from build123d import *

# Parameters (mm, degrees)
ESQUISSE1_W             = 43
ESQUISSE1_H             = 80
BOSS_EXTRU_1_DEPTH      = 5
ESQUISSE2_W             = 5
ESQUISSE2_H             = 80
BOSS_EXTRU_2_DEPTH      = 38.5
ENL_V_MAT_EXTRU_1_REACH = 84.692
ESQUISSE3_R             = 1.75
ESQUISSE4_W             = 5
ESQUISSE4_H             = 80
BOSS_EXTRU_3_DEPTH      = 20
ENL_V_MAT_EXTRU_2_REACH = 82.206
ESQUISSE5_R             = 2.75
ENL_V_MAT_EXTRU_3_REACH = 80.13
ESQUISSE6_R             = 1.5
BOSS_EXTRU_4_DEPTH      = 80
ENL_V_MAT_EXTRU_4_REACH = 82.206
ESQUISSE8_R             = 6
CHANFREIN2_SIZE         = 8.5
CHANFREIN2_SIZE2        = 10


with BuildPart() as part:
    # Esquisse1 → Boss.-Extru.1 (new body)
    with BuildSketch(Plane.XY):
        with Locations((-11.896872358, -15.648351648)):
            Rectangle(ESQUISSE1_W, ESQUISSE1_H)
    extrude(amount=BOSS_EXTRU_1_DEPTH)

    # Esquisse2 → Boss.-Extru.2 (add)
    with BuildSketch(Plane(origin=(0, 0, 5), x_dir=(-1, 0, 0), z_dir=(0, 0, -1))):
        with Locations((-7.103127642, -15.648351648)):
            Rectangle(ESQUISSE2_W, ESQUISSE2_H)
    extrude(amount=-BOSS_EXTRU_2_DEPTH)

    # Esquisse3 → Enlèv. mat.-Extru.1 (cut, up to next)
    with BuildSketch(Plane(origin=(9.603127642, 0, 0), x_dir=(0, 0, -1), z_dir=(1, 0, 0)), mode=Mode.PRIVATE) as enl_v_mat_extru_1_sk1:
        with Locations(Location((-40, -52.148351648, 0), (0, 0, 90))):
            Circle(ESQUISSE3_R)
    enl_v_mat_extru_1_tool1 = extrude(enl_v_mat_extru_1_sk1.sketch, amount=-ENL_V_MAT_EXTRU_1_REACH, mode=Mode.PRIVATE) & part.part
    # Esquisse3 → Enlèv. mat.-Extru.1 (cut, up to next)
    with BuildSketch(Plane(origin=(9.603127642, 0, 0), x_dir=(0, 0, -1), z_dir=(1, 0, 0)), mode=Mode.PRIVATE) as enl_v_mat_extru_1_sk2:
        with Locations(Location((-40, -32.148351648, 0), (0, 0, 90))):
            Circle(ESQUISSE3_R)
    enl_v_mat_extru_1_tool2 = extrude(enl_v_mat_extru_1_sk2.sketch, amount=-ENL_V_MAT_EXTRU_1_REACH, mode=Mode.PRIVATE) & part.part
    # Esquisse3 → Enlèv. mat.-Extru.1 (cut, up to next)
    with BuildSketch(Plane(origin=(9.603127642, 0, 0), x_dir=(0, 0, -1), z_dir=(1, 0, 0)), mode=Mode.PRIVATE) as enl_v_mat_extru_1_sk3:
        with Locations(Location((-20, -32.148351648, 0), (0, 0, 90))):
            Circle(ESQUISSE3_R)
    enl_v_mat_extru_1_tool3 = extrude(enl_v_mat_extru_1_sk3.sketch, amount=-ENL_V_MAT_EXTRU_1_REACH, mode=Mode.PRIVATE) & part.part
    # Esquisse3 → Enlèv. mat.-Extru.1 (cut, up to next)
    with BuildSketch(Plane(origin=(9.603127642, 0, 0), x_dir=(0, 0, -1), z_dir=(1, 0, 0)), mode=Mode.PRIVATE) as enl_v_mat_extru_1_sk4:
        with Locations(Location((-20, -52.148351648, 0), (0, 0, 90))):
            Circle(ESQUISSE3_R)
    enl_v_mat_extru_1_tool4 = extrude(enl_v_mat_extru_1_sk4.sketch, amount=-ENL_V_MAT_EXTRU_1_REACH, mode=Mode.PRIVATE) & part.part
    # Esquisse3 → Enlèv. mat.-Extru.1 (cut, up to next)
    with BuildSketch(Plane(origin=(9.603127642, 0, 0), x_dir=(0, 0, -1), z_dir=(1, 0, 0)), mode=Mode.PRIVATE) as enl_v_mat_extru_1_sk5:
        with Locations(Location((-40, 0.851648352, 0), (0, 0, 90))):
            Circle(ESQUISSE3_R)
    enl_v_mat_extru_1_tool5 = extrude(enl_v_mat_extru_1_sk5.sketch, amount=-ENL_V_MAT_EXTRU_1_REACH, mode=Mode.PRIVATE) & part.part
    # Esquisse3 → Enlèv. mat.-Extru.1 (cut, up to next)
    with BuildSketch(Plane(origin=(9.603127642, 0, 0), x_dir=(0, 0, -1), z_dir=(1, 0, 0)), mode=Mode.PRIVATE) as enl_v_mat_extru_1_sk6:
        with Locations(Location((-40, 20.851648352, 0), (0, 0, 90))):
            Circle(ESQUISSE3_R)
    enl_v_mat_extru_1_tool6 = extrude(enl_v_mat_extru_1_sk6.sketch, amount=-ENL_V_MAT_EXTRU_1_REACH, mode=Mode.PRIVATE) & part.part
    # Esquisse3 → Enlèv. mat.-Extru.1 (cut, up to next)
    with BuildSketch(Plane(origin=(9.603127642, 0, 0), x_dir=(0, 0, -1), z_dir=(1, 0, 0)), mode=Mode.PRIVATE) as enl_v_mat_extru_1_sk7:
        with Locations(Location((-20, 20.851648352, 0), (0, 0, 90))):
            Circle(ESQUISSE3_R)
    enl_v_mat_extru_1_tool7 = extrude(enl_v_mat_extru_1_sk7.sketch, amount=-ENL_V_MAT_EXTRU_1_REACH, mode=Mode.PRIVATE) & part.part
    # Esquisse3 → Enlèv. mat.-Extru.1 (cut, up to next)
    with BuildSketch(Plane(origin=(9.603127642, 0, 0), x_dir=(0, 0, -1), z_dir=(1, 0, 0)), mode=Mode.PRIVATE) as enl_v_mat_extru_1_sk8:
        with Locations(Location((-20, 0.851648352, 0), (0, 0, 90))):
            Circle(ESQUISSE3_R)
    enl_v_mat_extru_1_tool8 = extrude(enl_v_mat_extru_1_sk8.sketch, amount=-ENL_V_MAT_EXTRU_1_REACH, mode=Mode.PRIVATE) & part.part
    add(enl_v_mat_extru_1_tool1.solids().sort_by_distance((9.603128, -52.148352, 40))[0], mode=Mode.SUBTRACT)
    add(enl_v_mat_extru_1_tool2.solids().sort_by_distance((9.603128, -32.148352, 40))[0], mode=Mode.SUBTRACT)
    add(enl_v_mat_extru_1_tool3.solids().sort_by_distance((9.603128, -32.148352, 20))[0], mode=Mode.SUBTRACT)
    add(enl_v_mat_extru_1_tool4.solids().sort_by_distance((9.603128, -52.148352, 20))[0], mode=Mode.SUBTRACT)
    add(enl_v_mat_extru_1_tool5.solids().sort_by_distance((9.603128, 0.851648, 40))[0], mode=Mode.SUBTRACT)
    add(enl_v_mat_extru_1_tool6.solids().sort_by_distance((9.603128, 20.851648, 40))[0], mode=Mode.SUBTRACT)
    add(enl_v_mat_extru_1_tool7.solids().sort_by_distance((9.603128, 20.851648, 20))[0], mode=Mode.SUBTRACT)
    add(enl_v_mat_extru_1_tool8.solids().sort_by_distance((9.603128, 0.851648, 20))[0], mode=Mode.SUBTRACT)

    # Esquisse4 → Boss.-Extru.3 (add)
    with BuildSketch(Plane(origin=(0, 0, 0), x_dir=(-1, 0, 0), z_dir=(0, 0, -1))):
        with Locations((30.896872358, -15.648351648)):
            Rectangle(ESQUISSE4_W, ESQUISSE4_H)
    extrude(amount=BOSS_EXTRU_3_DEPTH)

    # Esquisse5 → Enlèv. mat.-Extru.2 (cut, up to next)
    with BuildSketch(Plane(origin=(-28.396872358, 0, 0), x_dir=(0, 0, -1), z_dir=(1, 0, 0)), mode=Mode.PRIVATE) as enl_v_mat_extru_2_sk1:
        with Locations(Location((10, 14.351648352, 0), (0, 0, 90))):
            Circle(ESQUISSE5_R)
    enl_v_mat_extru_2_tool1 = extrude(enl_v_mat_extru_2_sk1.sketch, amount=-ENL_V_MAT_EXTRU_2_REACH, mode=Mode.PRIVATE) & part.part
    # Esquisse5 → Enlèv. mat.-Extru.2 (cut, up to next)
    with BuildSketch(Plane(origin=(-28.396872358, 0, 0), x_dir=(0, 0, -1), z_dir=(1, 0, 0)), mode=Mode.PRIVATE) as enl_v_mat_extru_2_sk2:
        with Locations(Location((10, -5.648351648, 0), (0, 0, 90))):
            Circle(ESQUISSE5_R)
    enl_v_mat_extru_2_tool2 = extrude(enl_v_mat_extru_2_sk2.sketch, amount=-ENL_V_MAT_EXTRU_2_REACH, mode=Mode.PRIVATE) & part.part
    # Esquisse5 → Enlèv. mat.-Extru.2 (cut, up to next)
    with BuildSketch(Plane(origin=(-28.396872358, 0, 0), x_dir=(0, 0, -1), z_dir=(1, 0, 0)), mode=Mode.PRIVATE) as enl_v_mat_extru_2_sk3:
        with Locations(Location((10, -25.648351648, 0), (0, 0, 90))):
            Circle(ESQUISSE5_R)
    enl_v_mat_extru_2_tool3 = extrude(enl_v_mat_extru_2_sk3.sketch, amount=-ENL_V_MAT_EXTRU_2_REACH, mode=Mode.PRIVATE) & part.part
    # Esquisse5 → Enlèv. mat.-Extru.2 (cut, up to next)
    with BuildSketch(Plane(origin=(-28.396872358, 0, 0), x_dir=(0, 0, -1), z_dir=(1, 0, 0)), mode=Mode.PRIVATE) as enl_v_mat_extru_2_sk4:
        with Locations(Location((10, -45.648351648, 0), (0, 0, 90))):
            Circle(ESQUISSE5_R)
    enl_v_mat_extru_2_tool4 = extrude(enl_v_mat_extru_2_sk4.sketch, amount=-ENL_V_MAT_EXTRU_2_REACH, mode=Mode.PRIVATE) & part.part
    add(enl_v_mat_extru_2_tool1.solids().sort_by_distance((-28.396872, 14.351648, -10))[0], mode=Mode.SUBTRACT)
    add(enl_v_mat_extru_2_tool2.solids().sort_by_distance((-28.396872, -5.648352, -10))[0], mode=Mode.SUBTRACT)
    add(enl_v_mat_extru_2_tool3.solids().sort_by_distance((-28.396872, -25.648352, -10))[0], mode=Mode.SUBTRACT)
    add(enl_v_mat_extru_2_tool4.solids().sort_by_distance((-28.396872, -45.648352, -10))[0], mode=Mode.SUBTRACT)

    # Esquisse6 → Enlèv. mat.-Extru.3 (cut, up to next)
    with BuildSketch(Plane(origin=(0, 0, 0), x_dir=(-1, 0, 0), z_dir=(0, 0, -1)), mode=Mode.PRIVATE) as enl_v_mat_extru_3_sk1:
        with Locations((18.396872358, -45.648351648)):
            Circle(ESQUISSE6_R)
    enl_v_mat_extru_3_tool1 = extrude(enl_v_mat_extru_3_sk1.sketch, amount=-ENL_V_MAT_EXTRU_3_REACH, mode=Mode.PRIVATE) & part.part
    add(enl_v_mat_extru_3_tool1.solids().sort_by_distance((-18.396872, -45.648352, 0))[0], mode=Mode.SUBTRACT)

    # Esquisse7 → Boss.-Extru.4 (add)
    with BuildSketch(Plane(origin=(0, 24.351648352, 0), x_dir=(1, 0, 0), z_dir=(0, 1, 0))):
        Polygon((9.603127642, 0), (-28.396872358, 20), (-28.396872358, 14.349760381), (-1.132327635, 0), align=None)
    extrude(amount=-BOSS_EXTRU_4_DEPTH)

    # Enlèv. mat.-Extru.4: up to this plane
    enl_v_mat_extru_4_end = Plane(origin=(9.603127642, -98.590172756, 0), z_dir=(0.46574643283262246, 0, -0.8849182223819824))
    # Esquisse8 → Enlèv. mat.-Extru.4 (cut, up to the surface)
    with BuildSketch(Plane(origin=(-28.396872358, 0, 0), x_dir=(0, 0, -1), z_dir=(1, 0, 0)), mode=Mode.PRIVATE) as enl_v_mat_extru_4_sk1:
        with Locations(Location((10, -45.648351648, 0), (0, 0, 316.465525683))):
            Circle(ESQUISSE8_R)
    enl_v_mat_extru_4_tool1 = split(extrude(enl_v_mat_extru_4_sk1.sketch, amount=ENL_V_MAT_EXTRU_4_REACH, mode=Mode.PRIVATE), bisect_by=enl_v_mat_extru_4_end, keep=Keep.BOTH, mode=Mode.PRIVATE)
    add(enl_v_mat_extru_4_tool1.solids().sort_by_distance((-28.396872, -45.648352, -10))[0], mode=Mode.SUBTRACT)
    # Esquisse8 → Enlèv. mat.-Extru.4 (cut, up to the surface)
    with BuildSketch(Plane(origin=(-28.396872358, 0, 0), x_dir=(0, 0, -1), z_dir=(1, 0, 0)), mode=Mode.PRIVATE) as enl_v_mat_extru_4_sk2:
        with Locations(Location((10, -25.648351648, 0), (0, 0, 316.465525683))):
            Circle(ESQUISSE8_R)
    enl_v_mat_extru_4_tool2 = split(extrude(enl_v_mat_extru_4_sk2.sketch, amount=ENL_V_MAT_EXTRU_4_REACH, mode=Mode.PRIVATE), bisect_by=enl_v_mat_extru_4_end, keep=Keep.BOTH, mode=Mode.PRIVATE)
    add(enl_v_mat_extru_4_tool2.solids().sort_by_distance((-28.396872, -25.648352, -10))[0], mode=Mode.SUBTRACT)
    # Esquisse8 → Enlèv. mat.-Extru.4 (cut, up to the surface)
    with BuildSketch(Plane(origin=(-28.396872358, 0, 0), x_dir=(0, 0, -1), z_dir=(1, 0, 0)), mode=Mode.PRIVATE) as enl_v_mat_extru_4_sk3:
        with Locations(Location((10, -5.648351648, 0), (0, 0, 316.465525683))):
            Circle(ESQUISSE8_R)
    enl_v_mat_extru_4_tool3 = split(extrude(enl_v_mat_extru_4_sk3.sketch, amount=ENL_V_MAT_EXTRU_4_REACH, mode=Mode.PRIVATE), bisect_by=enl_v_mat_extru_4_end, keep=Keep.BOTH, mode=Mode.PRIVATE)
    add(enl_v_mat_extru_4_tool3.solids().sort_by_distance((-28.396872, -5.648352, -10))[0], mode=Mode.SUBTRACT)
    # Esquisse8 → Enlèv. mat.-Extru.4 (cut, up to the surface)
    with BuildSketch(Plane(origin=(-28.396872358, 0, 0), x_dir=(0, 0, -1), z_dir=(1, 0, 0)), mode=Mode.PRIVATE) as enl_v_mat_extru_4_sk4:
        with Locations(Location((10, 14.351648352, 0), (0, 0, 316.465525683))):
            Circle(ESQUISSE8_R)
    enl_v_mat_extru_4_tool4 = split(extrude(enl_v_mat_extru_4_sk4.sketch, amount=ENL_V_MAT_EXTRU_4_REACH, mode=Mode.PRIVATE), bisect_by=enl_v_mat_extru_4_end, keep=Keep.BOTH, mode=Mode.PRIVATE)
    add(enl_v_mat_extru_4_tool4.solids().sort_by_distance((-28.396872, 14.351648, -10))[0], mode=Mode.SUBTRACT)

    # Chanfrein2
    chanfrein2_edges = [part.edges().sort_by_distance(p)[0] for p in [
        (4.603127642, -15.648351648, 5),
    ]]
    chanfrein2_side = [part.faces().sort_by_distance(p)[0] for p in [
        (4.603127642, -15.648351648, 24.102624942),
    ]]
    chamfer(chanfrein2_edges, length=CHANFREIN2_SIZE, length2=CHANFREIN2_SIZE2, reference=chanfrein2_side[0])


solid = part.part
Source: CAD feature listing. Evaluate the final solid. Frame: model axes, mm. A direction names the side the tool comes from. Give positions to 0.01 mm unless a question says otherwise; leave off trailing zeros. Write each loop counter-clockwise with the first axis right and the second up, starting at its lowest first coordinate (ties: lowest second). Pieces come first, ordered by that corner, then holes. Notation, with made-up numbers: (70.5, -11) -> (98.5, -11) arc R8 ccw to (98.5, 1) -> close; hole circle Ø10 at (59.5, 31.25). An arc over 180 degrees is marked (long way). Return JSON: item names as keys, results as strings. Group by question number.
1. Section D-D, the plane x = -4.5. Output: boundary loops of the cut face in (y, z).
2. Pin query (flat end, axial travel): pin 1 Ø8 at (x, y) = (-8.5, 1.5) entering from -Z; pin 2 Ø3.5 at (y, z) = (-25.65, -10) entering from +X; pin 3 Ø8 at (y, z) = (-19.5, 14) entering from -X; pin 4 Ø6.5 at (y, z) = (-45.65, -10) entering from +X. Return the tip coordinate at first contact, or that it passes through.
3. Section A-A, the plane z = 40. Output: boundary loops of the cut face in (x, y).
4. Mould query, pull axis Z, two halves, no side actions, for faces 4 (the face through (7.14, 19.56, 21.18)), 5 (the face through (7.14, -51.34, 38.45)), 6 (the face through (-20, -15, 5)), 7 (the face through (-31, -15, -20)). Classes: +Z half, -Z half, draft (parallel to the pull), parting line (faces both ways), or undercut.
5. Access query for faces 1 (the face through (-15, -15, 0)), 2 (the face through (-12.97, -10.96, -7.21)), 3 (the face through (4.603, -16, 28)). Directions: +Z, -Z, +X, -X, +Y, -Y. A direction counts if a zero-diameter tool reaches every point of the face in a straight line with its end or side. Return the directions, or none.
6. Material intervals for line 1 (X direction, y = 2, z = 26.5); line 2 (Z direction, x = -5, y = -48.5); line 3 (Z direction, x = -27.5, y = -9.5), sorted ascending. Write a range as from..to.
7. Section B-B, the plane y = -38. Output: boundary loops of the cut face in (x, z).
8. Section C-C, the plane x = -12. Output: boundary loops of the cut face in (y, z), then the cut area to 3 significant figures.
Determined:
{
 "1": {"outline": "(-55.65, -7.42) -> (-51.07, -7.42) arc R6 cw to (-40.23, -7.42) -> (-31.07, -7.42) arc R6 cw to (-20.23, -7.42) -> (-11.07, -7.42) arc R6 cw to (-0.23, -7.42) -> (8.93, -7.42) arc R6 cw to (19.77, -7.42) -> (24.35, -7.42) -> (24.35, -1.77) -> (-55.65, -1.77) -> close; (-55.65, 0) -> (24.35, 0) -> (24.35, 5.76) -> (-55.65, 5.76) -> close"},
 "2": {"pin 1": "stops at z = -11.63", "pin 2": "passes through", "pin 3": "stops at x = 0.49", "pin 4": "stops at x = -28.4"},
 "3": {"outline": "(4.6, -55.65) -> (9.6, -55.65) -> (9.6, -53.9) -> (4.6, -53.9) -> close; (4.6, -50.4) -> (9.6, -50.4) -> (9.6, -33.9) -> (4.6, -33.9) -> close; (4.6, -30.4) -> (9.6, -30.4) -> (9.6, -0.9) -> (4.6, -0.9) -> close; (4.6, 2.6) -> (9.6, 2.6) -> (9.6, 19.1) -> (4.6, 19.1) -> close; (4.6, 22.6) -> (9.6, 22.6) -> (9.6, 24.35) -> (4.6, 24.35) -> close"},
 "4": {"face 4": "undercut", "face 5": "undercut", "face 6": "+Z half", "face 7": "-Z half"},
 "5": {"face 1": "+Y, -Y", "face 2": "+X", "face 3": "+Z, -X, +Y, -Y"},
 "6": {"line 1": "x = 4.6..9.6", "line 2": "z = -4.72..-2.04, 0..5.34", "line 3": "z = -19.53..-14.6, 0..5"},
 "7": {"outline": "(-33.4, -20) -> (-28.4, -20) -> (9.6, 0) -> (9.6, 43.5) -> (4.6, 43.5) -> (4.6, 13.5) -> (-5.4, 5) -> (-33.4, 5) -> close; hole (-28.4, -14.35) -> (-1.13, 0) -> (-28.4, 0) -> close"},
 "8": {"outline": "(-55.65, -11.37) -> (-51.49, -11.37) arc R6 cw to (-49.85, -5.72) -> (-55.65, -5.72) -> close; (-55.65, 0) -> (24.35, 0) -> (24.35, 5) -> (-55.65, 5) -> close; (-41.44, -5.72) arc R6 cw to (-39.81, -11.37) -> (-31.49, -11.37) arc R6 cw to (-29.85, -5.72) -> close; (-21.44, -5.72) arc R6 cw to (-19.81, -11.37) -> (-11.49, -11.37) arc R6 cw to (-9.85, -5.72) -> close; (-1.44, -5.72) arc R6 cw to (0.19, -11.37) -> (8.51, -11.37) arc R6 cw to (10.15, -5.72) -> close; (18.56, -5.72) arc R6 cw to (20.19, -11.37) -> (24.35, -11.37) -> (24.35, -5.72) -> close", "area": "600 mm2"}
}
